from build123d import *

# Parameters (mm, degrees)
SKETCH1_R               = 22.5
SKETCH1_R_2             = 17.5
BOSS_EXTRUDE1_DEPTH     = 20
BOSS_EXTRUDE5_DEPTH     = 20
BOSS_EXTRUDE5_2_DEPTH   = 20
SKETCH5_W               = 70
SKETCH5_H               = 60.378075934
BOSS_EXTRUDE7_DEPTH     = 5
SKETCH6_W               = 15
SKETCH6_H               = 5
SKETCH6_W_2             = 52.6
SKETCH6_H_2             = 21
BOSS_EXTRUDE8_DEPTH     = 40
SKETCH7_W               = 100
SKETCH7_H               = 31
BOSS_EXTRUDE9_DEPTH     = 5
CUT_EXTRUDE1_DEPTH      = 1
CUT_EXTRUDE1_DEPTH_BACK = 66
FILLET1_R               = 30
SKETCH9_W               = 30
SKETCH9_H               = 31
BOSS_EXTRUDE10_DEPTH    = 5
SKETCH10_R              = 3.5
CUT_EXTRUDE2_DEPTH      = 71
SKETCH11_R              = 12.5
CUT_EXTRUDE3_DEPTH      = 45
SKETCH12_R              = 3.5
CUT_EXTRUDE4_DEPTH      = 61.378075935


with BuildPart() as part:
    # Sketch1 → Boss-Extrude1 (new body)
    with BuildSketch(Plane(origin=(0, 0, 0), x_dir=(1, 0, 0), z_dir=(0, 1, 0))):
        Circle(SKETCH1_R)
        Circle(SKETCH1_R_2, mode=Mode.SUBTRACT)
    extrude(amount=BOSS_EXTRUDE1_DEPTH)



with BuildPart() as body_2:
    # Sketch2 → Boss-Extrude5 (new body)
    with BuildSketch(Plane(origin=(0, 20, 0), x_dir=(1, 0, 0), z_dir=(0, 1, 0))):
        with BuildLine():
            Line((-20.566963801, -19), (-30, -19))
            Line((-30, -19), (-30, -30.189037967))
            Line((-30, -30.189037967), (30, -30.189037967))
            Line((30, -30.189037967), (30, -19))
            Line((30, -19), (20.566963801, -19))
            ThreePointArc((20.566963801, -19), (0, -28), (-20.566963801, -19))
        make_face()
    extrude(amount=-BOSS_EXTRUDE5_DEPTH)


with BuildPart() as body_3:
    # Sketch2 → Boss-Extrude5 2 (new body)
    with BuildSketch(Plane(origin=(0, 20, 0), x_dir=(1, 0, 0), z_dir=(0, 1, 0))):
        with BuildLine():
            Line((-30, 30.189037967), (-30, 19))
            Line((-30, 19), (-20.566963801, 19))
            ThreePointArc((-20.566963801, 19), (0, 28), (20.566963801, 19))
            Line((20.566963801, 19), (30, 19))
            Line((30, 19), (30, 30.189037967))
            Line((30, 30.189037967), (-30, 30.189037967))
        make_face()
    extrude(amount=-BOSS_EXTRUDE5_2_DEPTH)


with BuildPart() as part_1:
    add(part.part)

    add(body_2.part)  # Boss-Extrude7 merges body 2

    add(body_3.part)  # Boss-Extrude7 merges body 3
    # Sketch5 → Boss-Extrude7 (add)
    with BuildSketch(Plane(origin=(0, 20, 0), x_dir=(1, 0, 0), z_dir=(0, 1, 0))):
        Rectangle(SKETCH5_W, SKETCH5_H)
    extrude(amount=BOSS_EXTRUDE7_DEPTH)

    # Sketch6 → Boss-Extrude8 (add)
    with BuildSketch(Plane(origin=(0, 25, 0), x_dir=(1, 0, 0), z_dir=(0, 1, 0))):
        Polygon((26.3, -10.5), (-26.3, -10.5), (-35, -10.5), (-35, -15.5), (35, -15.5), (35, -10.5), align=None)
        with Locations((42.5, -13)):
            Rectangle(SKETCH6_W, SKETCH6_H)
        with Locations((-42.5, -13)):
            Rectangle(SKETCH6_W, SKETCH6_H)
        with Locations((-42.5, 13)):
            Rectangle(SKETCH6_W, SKETCH6_H)
        Polygon((-35, 10.5), (-26.3, 10.5), (26.3, 10.5), (35, 10.5), (35, 15.5), (-35, 15.5), align=None)
        with Locations((42.5, 13)):
            Rectangle(SKETCH6_W, SKETCH6_H)
        Rectangle(SKETCH6_W_2, SKETCH6_H_2)
    extrude(amount=BOSS_EXTRUDE8_DEPTH)

    # Sketch7 → Boss-Extrude9 (add)
    with BuildSketch(Plane.XZ.offset(-25)):
        Rectangle(SKETCH7_W, SKETCH7_H)
    extrude(amount=BOSS_EXTRUDE9_DEPTH)

    # Sketch8 → Cut-Extrude1 (cut, two sides)
    with BuildSketch(Plane.XZ) as cut_extrude1_sk:
        with BuildLine():
            ThreePointArc((48.319407886, 15.5), (0, 50.744607383), (-48.319407886, 15.5))
            Line((-48.319407886, 15.5), (-35, 15.5))
            ThreePointArc((-35, 15.5), (0, 38.278584091), (35, 15.5))
            Line((35, 15.5), (48.319407886, 15.5))
        make_face()
        with BuildLine():
            Line((-35, -15.5), (-48.319407886, -15.5))
            ThreePointArc((-48.319407886, -15.5), (0, -50.744607383), (48.319407886, -15.5))
            Line((48.319407886, -15.5), (35, -15.5))
            ThreePointArc((35, -15.5), (0, -38.278584091), (-35, -15.5))
        make_face()
    extrude(amount=CUT_EXTRUDE1_DEPTH, mode=Mode.SUBTRACT)
    extrude(cut_extrude1_sk.sketch, amount=-CUT_EXTRUDE1_DEPTH_BACK, mode=Mode.SUBTRACT)

    # Fillet1
    fillet1_edges = [part_1.edges().sort_by_distance(p)[0] for p in [
        (-50, 65, -13),
        (50, 65, 13),
    ]]
    fillet(fillet1_edges, radius=FILLET1_R)

    # Sketch9 → Boss-Extrude10 (add)
    with BuildSketch(Plane(origin=(0, 65, 0), x_dir=(1, 0, 0), z_dir=(0, 1, 0))):
        Rectangle(SKETCH9_W, SKETCH9_H)
    extrude(amount=BOSS_EXTRUDE10_DEPTH)

    # Sketch10 → Cut-Extrude2 (cut, through all)
    with BuildSketch(Plane(origin=(0, 70, 0), x_dir=(1, 0, 0), z_dir=(0, 1, 0))):
        Circle(SKETCH10_R)
    extrude(amount=-CUT_EXTRUDE2_DEPTH, mode=Mode.SUBTRACT)

    # Sketch11 → Cut-Extrude3 (cut)
    with BuildSketch(Plane.XZ.offset(-20)):
        Circle(SKETCH11_R)
    extrude(amount=-CUT_EXTRUDE3_DEPTH, mode=Mode.SUBTRACT)

    # Sketch12 → Cut-Extrude4 (cut, through all)
    with BuildSketch(Plane.XY.offset(30.189037967)):
        with Locations((0, 12.5)):
            Circle(SKETCH12_R)
    extrude(amount=-CUT_EXTRUDE4_DEPTH, mode=Mode.SUBTRACT)


solid = part_1.part
Build history of the part. All positions in model axes, mm. A direction names the side the tool comes from. Give positions to 0.01 mm unless a question says otherwise; leave off trailing zeros. Order: outer loops, then holes, each group sorted by start corner. A loop starts at its lowest first (then second) coordinate and runs counter-clockwise, first axis right, second up. Notation, with made-up numbers: M 77,81 L 83,81 A33 ccw 83,114 Z; hole C 37.25,30 d5. An arc over 180 degrees is marked long. Put each result on its own line as item: value.
Item 1: Wall check: probe 1 along Y at (x, z) = (0, -18.65); probe 2 along Z at (x, y) = (0, 39); probe 3 along Z at (x, y) = (-7, 7). Give the ranges that are in metal, low to high.
Results are:
probe 1: 0 to 9, 16 to 25
probe 2: -15.5 to -12.5, 12.5 to 15.5
probe 3: -30.19 to -27.11, -21.38 to -16.04, 16.04 to 21.38, 27.11 to 30.19
Item 2: Which spindle directions (+Z, -Z, +X, -X, +Y, -Y) get a long thin tool onto all of the face, cutting with end or side? Do faces 1 (the face through (0, 8, 28)), 2 (the face through (-35, 40, 10.5)), 3 (the face through (-30, 10, -21)). Say none if no direction does.
Results are:
face 1: -Y
face 2: -X, +Y
face 3: +Z, -Z, -X, -Y
Item 3: Cut at D-D on x = 38.5. Write the cut outline in (y, z).
Results are:
outline: M 20,-15.5 L 58.62,-15.5 L 58.62,-10.5 L 25,-10.5 L 25,10.5 L 58.62,10.5 L 58.62,15.5 L 20,15.5 Z
Item 4: Cut at A-A on y = 7.5. Write the cut outline in (x, z), then the cut area to 3 significant figures.
Results are:
outline: M -30,-23.77 A38.28 ccw -23.53,-30.19 L 23.53,-30.19 A38.28 ccw 30,-23.77 L 30,-19 L 20.57,-19 A28 cw -20.57,-19 L -30,-19 Z; M -30,19 L -20.57,19 A28 cw 20.57,19 L 30,19 L 30,23.77 A38.28 ccw 23.53,30.19 L -23.53,30.19 A38.28 ccw -30,23.77 Z; C 0,0 d45; hole C 0,0 d35
area: 1,380 mm2
Item 5: Drop flat-ended pins along their axis: pin 1 Ø1.5 at (x, y) = (-33.5, 57.5) entering from -Z; pin 2 Ø10.5 at (x, z) = (-38.5, -3) entering from +Y; pin 3 Ø5 at (y, z) = (44, 17) entering from -X; pin 4 Ø3 at (x, z) = (33.5, 23.5) entering from -Y. Give the stop position or say it passes through.
Results are:
pin 1: z = -15.5
pin 2: y = 25
pin 3: x = -49.17
pin 4: through
Item 6: Pull direction X, two halves, no side cores. Call faces 4 (the face through (-3.497, 12.654, -28.967)), 5 (the face through (-15, 67, 0)), 6 (the face through (-3.497, 12.654, 29.001)), 7 (the face through (-38, 25, 0)): +X half, -X half, draft (parallel to the pull), parting line (faces both ways), or undercut.
Results are:
face 4: undercut
face 5: -X half
face 6: undercut
face 7: draft
Item 7: Cut at C-C on y = 32.5. Write the cut outline in (x, z).
Results are:
outline: M -50,-15.5 L 50,-15.5 L 50,-10.5 L 26.3,-10.5 L 26.3,10.5 L 50,10.5 L 50,15.5 L -50,15.5 L -50,10.5 L -26.3,10.5 L -26.3,-10.5 L -50,-10.5 Z; hole C 0,0 d25
